from build123d import *

# Parameters (mm, degrees)
SKETCH3_R               = 140
BOSS_EXTRUDE1_DEPTH     = 225
SKETCH4_R               = 97
CUT_EXTRUDE1_DEPTH      = 300.708191413
BOSS_EXTRUDE3_DEPTH     = 32
SKETCH11_R              = 23.5
CUT_EXTRUDE3_DEPTH      = 348.634865915
CIRPATTERN15_COUNT      = 3
MIRROR6_COPY_1_DEPTH    = 32
MIRROR6_COPY_2_DEPTH    = 32
MIRROR6_COPY_3_SKETCH_R = 23.5
MIRROR6_COPY_3_DEPTH    = 348.634865915
MIRROR6_COPY_4_SKETCH_R = 23.5
MIRROR6_COPY_4_DEPTH    = 348.634865915
SKETCH16_R              = 100
BOSS_EXTRUDE4_DEPTH     = 160
SKETCH17_R              = 50
CUT_EXTRUDE4_DEPTH      = 25
SKETCH18_R              = 28
CUT_EXTRUDE5_DEPTH      = 470.945948606
SKETCH19_R              = 12
CUT_EXTRUDE6_DEPTH      = 15
SKETCH20_R              = 97
CUT_EXTRUDE7_DEPTH      = 377.661910221


with BuildPart() as part:
    # Sketch3 → Boss-Extrude1 (new body)
    with BuildSketch(Plane(origin=(0, 0, 0), x_dir=(1, 0, 0), z_dir=(0, 1, 0))):
        with Locations(Location((0, 0, 0), (0, 0, 270))):
            Circle(SKETCH3_R)
    extrude(amount=BOSS_EXTRUDE1_DEPTH)

    # Sketch4 → Cut-Extrude1 (cut, through all)
    with BuildSketch(Plane.XZ):
        with Locations(Location((0, 0, 0), (0, 0, 270))):
            Circle(SKETCH4_R)
    extrude(amount=-CUT_EXTRUDE1_DEPTH, mode=Mode.SUBTRACT)

    # Sketch10 → Boss-Extrude3 (add)
    with BuildSketch(Plane.XZ):
        with BuildLine():
            Line((-50, 175), (-50, 130.766968306))
            ThreePointArc((-50, 130.766968306), (0, 140), (50, 130.766968306))
            Line((50, 130.766968306), (50, 175))
            ThreePointArc((50, 175), (0, 225), (-50, 175))
        make_face()
    boss_extrude3 = extrude(amount=-BOSS_EXTRUDE3_DEPTH)

    # Sketch11 → Cut-Extrude3 (cut, through all)
    with BuildSketch(Plane.XZ):
        with Locations(Location((0, 175, 0), (0, 0, 270))):
            Circle(SKETCH11_R)
    cut_extrude3 = extrude(amount=-CUT_EXTRUDE3_DEPTH, mode=Mode.SUBTRACT)

    # CirPattern15: Boss-Extrude3, Cut-Extrude3 ×3 about axis
    cirpattern15_axis = Axis((0, 0, 0), (0, 1, 0))
    add([boss_extrude3.rotate(cirpattern15_axis, i * 360 / CIRPATTERN15_COUNT) for i in range(1, CIRPATTERN15_COUNT)])
    add([cut_extrude3.rotate(cirpattern15_axis, i * 360 / CIRPATTERN15_COUNT) for i in range(1, CIRPATTERN15_COUNT)], mode=Mode.SUBTRACT)

    # Mirror6: Boss-Extrude3, Cut-Extrude3 across plane
    add(boss_extrude3.mirror(Plane.ZX.offset(112.5)))
    add(cut_extrude3.mirror(Plane.ZX.offset(112.5)), mode=Mode.SUBTRACT)

    # Mirror6 copy 1 sketch → Mirror6 copy 1 (add)
    with BuildSketch(Plane(origin=(0, 225, 0), x_dir=(-0.4999999999999998, 0, -0.8660254037844387), z_dir=(0, 1, 0))):
        with BuildLine():
            Line((-50, -175), (-50, -130.766968306))
            ThreePointArc((-50, -130.766968306), (0, -140), (50, -130.766968306))
            Line((50, -130.766968306), (50, -175))
            ThreePointArc((50, -175), (0, -225), (-50, -175))
        make_face()
    extrude(amount=-MIRROR6_COPY_1_DEPTH)

    # Mirror6 copy 2 sketch → Mirror6 copy 2 (add)
    with BuildSketch(Plane(origin=(0, 225, 0), x_dir=(-0.5000000000000004, 0, 0.8660254037844384), z_dir=(0, 1, 0))):
        with BuildLine():
            Line((-50, -175), (-50, -130.766968306))
            ThreePointArc((-50, -130.766968306), (0, -140), (50, -130.766968306))
            Line((50, -130.766968306), (50, -175))
            ThreePointArc((50, -175), (0, -225), (-50, -175))
        make_face()
    extrude(amount=-MIRROR6_COPY_2_DEPTH)

    # Mirror6 copy 3 sketch → Mirror6 copy 3 (cut, through all)
    with BuildSketch(Plane(origin=(0, 225, 0), x_dir=(-0.4999999999999998, 0, -0.8660254037844387), z_dir=(0, 1, 0))):
        with Locations((0, -175)):
            Circle(MIRROR6_COPY_3_SKETCH_R)
    extrude(amount=-MIRROR6_COPY_3_DEPTH, mode=Mode.SUBTRACT)

    # Mirror6 copy 4 sketch → Mirror6 copy 4 (cut, through all)
    with BuildSketch(Plane(origin=(0, 225, 0), x_dir=(-0.5000000000000004, 0, 0.8660254037844384), z_dir=(0, 1, 0))):
        with Locations((0, -175)):
            Circle(MIRROR6_COPY_4_SKETCH_R)
    extrude(amount=-MIRROR6_COPY_4_DEPTH, mode=Mode.SUBTRACT)

    # Sketch16 → Boss-Extrude4 (add)
    with BuildSketch(Plane.XY):
        with Locations((0, 112.5)):
            Circle(SKETCH16_R)
    extrude(amount=-BOSS_EXTRUDE4_DEPTH)

    # Sketch17 → Cut-Extrude4 (cut)
    with BuildSketch(Plane(origin=(0, 0, -160), x_dir=(-1, 0, 0), z_dir=(0, 0, -1))):
        with Locations((0, 112.5)):
            Circle(SKETCH17_R)
    extrude(amount=-CUT_EXTRUDE4_DEPTH, mode=Mode.SUBTRACT)

    # Sketch18 → Cut-Extrude5 (cut, through all)
    with BuildSketch(Plane(origin=(0, 0, -135), x_dir=(-1, 0, 0), z_dir=(0, 0, -1))):
        with Locations((0, 112.5)):
            Circle(SKETCH18_R)
    extrude(amount=-CUT_EXTRUDE5_DEPTH, mode=Mode.SUBTRACT)

    # Sketch19 → Cut-Extrude6 (cut)
    with BuildSketch(Plane(origin=(0, 0, -160), x_dir=(-1, 0, 0), z_dir=(0, 0, -1))):
        with Locations((0, 187.5)):
            Circle(SKETCH19_R)
        with Locations((64.951905284, 75)):
            Circle(SKETCH19_R)
        with Locations((-64.951905284, 75)):
            Circle(SKETCH19_R)
    extrude(amount=-CUT_EXTRUDE6_DEPTH, mode=Mode.SUBTRACT)

    # Sketch20 → Cut-Extrude7 (cut, through all)
    with BuildSketch(Plane.XZ):
        with Locations(Location((0, 0, 0), (0, 0, 270))):
            Circle(SKETCH20_R)
    extrude(amount=-CUT_EXTRUDE7_DEPTH, mode=Mode.SUBTRACT)


solid = part.part
The model under review builds one solid part; all positions refer to its coordinate system, in mm. A direction names the side the tool comes from. Round coordinates to 2 decimals unless told otherwise and drop trailing zeros. Write each loop counter-clockwise with the first axis right and the second up, starting at its lowest first coordinate (ties: lowest second). Pieces come first, ordered by that corner, then holes. Notation, with made-up numbers: M 4,3 L 28,3 A32 cw 28,34 Z; hole C 51,31 d11. An arc over 180 degrees is marked long. Use a Markdown table: item, result. Add a question column.
Q1. Machinability: for faces 1 (the face through (-172, 32, -100)), 2 (the face through (50, 16, 153)), 3 (the face through (-23.07, 68.14, -147.68)), 4 (the face through (42.052, 110.925, 133.535)), which of the approach directions +Z, -Z, +X, -X, +Y, -Y give a long, thin tool a straight path to every point of the face, cutting with its end or side? Answer none if there is none.
Q2. We need section C-C, the plane y = 120. State the section outline as (x, z) points.
Q3. The part is to be moulded in two halves that separate along Z. For faces 5 (the face through (173, 32, -99)), 6 (the face through (-170.203, 209.224, -73.201)), 7 (the face through (-107.67, 15.78, -119.9)), say which applies: pulls with the +Z half, pulls with the -Z half, needs draft (parallel to the pull), parting line crosses it, or undercut.
Q4. We need section D-D, the plane z = -88. Count the separate pieces of the cut face and the enclosed holes in it, plus the area to 3 significant figures.
Q5. Insertion check: pin 1 (3 mm diameter, centred on y = 47, z = -98, fed in from +X); pin 2 (9.5 mm diameter, centred on y = 19, z = 159.5, fed in from +X); pin 3 (8 mm diameter, centred on x = 154.5, y = 202, fed in from -Z). Each pin has a flat end and moves straight along its axis. Give the tip position at first contact, or say it passes through.
Q6. To check wall thickness, follow line 1 (Y direction, x = -46.5, z = 190); line 2 (X direction, y = 19, z = -116.5); line 3 (X direction, y = 24.5, z = -67.5). State the ranges of each line that lie inside material, in increasing order.
Q7. We need section A-A, the plane z = 0. State the section outline as (x, y) points, plus the area to 4 significant figures.
Q8. We need section B-B, the plane x = 153.5. State the section outline as (y, z) points.
Findings below:
| question | item | result |
|---|---|---|
| 1 | face 1 | -Z, -X |
| 1 | face 2 | +Z, +X, +Y, -Y |
| 1 | face 3 | -Z |
| 1 | face 4 | none |
| 2 | outline | M -99.72,-160 L -49.43,-160 L -49.43,-135 L -26.98,-135 L -26.98,-93.17 A97 cw -26.98,93.17 L -26.98,137.38 A140 ccw -99.72,-98.27 Z; M 26.98,-135 L 49.43,-135 L 49.43,-160 L 99.72,-160 L 99.72,-98.27 A140 ccw 26.98,137.38 L 26.98,93.17 A97 cw 26.98,-93.17 Z |
| 3 | face 5 | needs draft |
| 3 | face 6 | undercut |
| 3 | face 7 | pulls with the -Z half |
| 4 | separate pieces | 6 |
| 4 | enclosed holes | 0 |
| 4 | area | 36,500 mm² |
| 5 | pin 1 | stops at x = 101.43 |
| 5 | pin 2 | stops at x = 50 |
| 5 | pin 3 | stops at z = -137.5 |
| 6 | line 1 | y = 0 to 32, 193 to 225 |
| 6 | line 2 | x = -192.29 to -101.78, -77.64 to 77.64, 101.78 to 192.29 |
| 6 | line 3 | x = -197.38 to -163.89, -139.22 to -69.66, 69.66 to 139.22, 163.89 to 197.38 |
| 7 | outline | M -140,0 L -97,0 L -97,225 L -140,225 Z; M 97,0 L 140,0 L 140,225 L 97,225 Z |
| 7 | area | 19,350 mm² |
| 8 | outline | M 0,-137.46 L 32,-137.46 L 32,-110.92 L 0,-110.92 Z; M 0,-64.08 L 32,-64.08 L 32,-30.89 L 0,-30.89 Z; M 193,-137.46 L 225,-137.46 L 225,-110.92 L 193,-110.92 Z; M 193,-64.08 L 225,-64.08 L 225,-30.89 L 193,-30.89 Z |
